Source: CAD feature listing. Evaluate the final solid. Frame: model axes, mm. A direction names the side the tool comes from. Round coordinates to 2 decimals unless told otherwise and drop trailing zeros. Write each loop counter-clockwise with the first axis right and the second up, starting at its lowest first coordinate (ties: lowest second). Pieces come first, ordered by that corner, then holes.
```python
from build123d import *


with BuildPart() as f2:
    # F2: sweep along a path in F1
    with BuildLine(Plane.XY) as f2_path:
        Line((0, 0), (-1056, 0))
        Line((-1056, 0), (-1056, 1962))
        Line((-1056, 1962), (-40, 1962))
    # F0 (on Right) → F2 (sweep)
    with BuildSketch(Plane.YZ):
        with BuildLine():
            ThreePointArc((15, 5), (13.5355339059, 8.5355339059), (10, 10))
            Line((10, 10), (-10, 10))
            ThreePointArc((-10, 10), (-13.5355339059, 8.5355339059), (-15, 5))
            Line((-15, 5), (-15, -5))
            ThreePointArc((-15, -5), (-13.5355339059, -8.5355339059), (-10, -10))
            Line((-10, -10), (10, -10))
            ThreePointArc((10, -10), (13.5355339059, -8.5355339059), (15, -5))
            Line((15, -5), (15, 5))
        make_face()
        with BuildLine():
            ThreePointArc((10, 9), (12.8284271247, 7.8284271247), (14, 5))
            Line((14, 5), (14, -5))
            ThreePointArc((14, -5), (12.8284271247, -7.8284271247), (10, -9))
            Line((10, -9), (-10, -9))
            ThreePointArc((-10, -9), (-12.8284271247, -7.8284271247), (-14, -5))
            Line((-14, -5), (-14, 5))
            ThreePointArc((-14, 5), (-12.8284271247, 7.8284271247), (-10, 9))
            Line((-10, 9), (10, 9))
        make_face(mode=Mode.SUBTRACT)
    sweep(path=f2_path.line, transition=Transition.RIGHT)


solid = f2.part
```
Q1. Set-up query: faces 1 (the face through (-1049, 986, 10)), 2 (the face through (-1049, 986, -9)). Return all of +Z, -Z, +X, -X, +Y, -Y with unobstructed straight access to the full face (end or side cutting, diameter ignored); none if empty.
Q2. Line query: line 1 (Y direction, x = -451.5, z = -2.5); line 2 (X direction, y = 1458.5, z = -4.25); line 3 (Y direction, x = -468.5, z = -5.75). Output: solid intervals per line, ascending.
Q3. Pin query (flat end, axial travel): P1, Ø10, axis at x = -952, z = -6.5, coming from the -Y side; P2, Ø1.5, axis at y = 1042.5, z = -3, coming from the +X side. Return the tip coordinate at first contact, or that it passes through.
Q4. Section query C-C, the plane z = -1.75. Output: boundary loops of the cut face in (x, y).
Q5. Section query B-B, the plane y = 533. Output: boundary loops of the cut face in (x, z).
Q6. Mould query, pull axis X, two halves, no side actions, for faces 3 (the face through (-1049, 976, 9)), 4 (the face through (-1049, 976, -10)). Classes: pulls with the +X half, pulls with the -X half, needs draft (parallel to the pull), parting line crosses it, or undercut.
Q7. Section query A-A, the plane x = -988. Give the number of separate pieces and of enclosed holes in the cut face, and give its area (3 significant figures).
Filled in:
1. face 1: +Z, +X, -X, +Y, -Y
1. face 2: none
2. line 1: y = -15 to -14, 14 to 15, 1947 to 1948, 1976 to 1977
2. line 2: x = -1071 to -1070, -1042 to -1041
2. line 3: y = -14.94 to -13.93, 13.93 to 14.94, 1947.06 to 1948.07, 1975.93 to 1976.94
3. P1: stops at y = -15
3. P2: stops at x = -1041
4. outline: (-1071, -15) - (0, -15) - (0, -14) - (-1070, -14) - (-1070, 1976) - (-40, 1976) - (-40, 1977) - (-1071, 1977) - close; (-1042, 14) - (0, 14) - (0, 15) - (-1041, 15) - (-1041, 1947) - (-40, 1947) - (-40, 1948) - (-1042, 1948) - close
5. outline: (-1071, -5) arc R5 ccw to (-1066, -10) - (-1046, -10) arc R5 ccw to (-1041, -5) - (-1041, 5) arc R5 ccw to (-1046, 10) - (-1066, 10) arc R5 ccw to (-1071, 5) - close; hole (-1070, -5) arc R4 ccw to (-1066, -9) - (-1046, -9) arc R4 ccw to (-1042, -5) - (-1042, 5) arc R4 ccw to (-1046, 9) - (-1066, 9) arc R4 ccw to (-1070, 5) - close
6. face 3: undercut
6. face 4: needs draft
7. separate pieces: 2
7. enclosed holes: 2
7. area: 177 mm2
